Geometry: final body of the model. Coordinates: model frame, mm. Coordinates: 2 decimals unless noted, no trailing zeros. Order: outer loops, then holes, each group sorted by start corner. A loop starts at its lowest first (then second) coordinate and runs counter-clockwise, first axis right, second up. Notation, with made-up numbers: M 62,75.25 L 66,75.25 A24 cw 66,97.25 Z; hole C 80,67.25 d11. An arc over 180 degrees is marked long. One line per question, with ' | ' between items.
from build123d import *

# Parameters (mm, degrees)
F0_W     = 30
F0_H     = 34
F0_R     = 1.575
F1_DEPTH = 4.826
F2_R     = 5


with BuildPart() as f1:
    # F0 (on Top) → F1 (new body)
    with BuildSketch(Plane.XY):
        Rectangle(F0_W, F0_H)
        with Locations((-8.8, -10)):
            Circle(F0_R, mode=Mode.SUBTRACT)
        with Locations((8.8, -10)):
            Circle(F0_R, mode=Mode.SUBTRACT)
        with Locations((-8.8, 10)):
            Circle(F0_R, mode=Mode.SUBTRACT)
        with Locations((8.8, 10)):
            Circle(F0_R, mode=Mode.SUBTRACT)
    extrude(amount=F1_DEPTH)

    # F2
    f2_edges = [f1.edges().sort_by_distance(p)[0] for p in [
        (-15, -17, 2.413),
        (15, -17, 2.413),
        (-15, 17, 2.413),
        (15, 17, 2.413),
    ]]
    fillet(f2_edges, radius=F2_R)


solid = f1.part
1. Draft query along Y for faces 1 (the face through (10.255, 9.397, 2.379)), 2 (the face through (13, -16, 2)), 3 (the face through (15, 0, 2)). Return one class per face: pulls with the +Y half, pulls with the -Y half, needs draft (parallel to the pull), parting line crosses it, or undercut.
Response values:
face 1: undercut | face 2: pulls with the -Y half | face 3: needs draft
2. Section B-B, the plane y = 11. Output: boundary loops of the cut face in (x, z).
Response values:
outline: M -15,0 L -10.02,0 L -10.02,4.83 L -15,4.83 Z; M -7.58,0 L 7.58,0 L 7.58,4.83 L -7.58,4.83 Z; M 10.02,0 L 15,0 L 15,4.83 L 10.02,4.83 Z
3. Section A-A, the plane z = 1.7. Output: boundary loops of the cut face in (x, y) (3 decimals).
Response values:
outline: M -15,-12 A5 ccw -10,-17 L 10,-17 A5 ccw 15,-12 L 15,12 A5 ccw 10,17 L -10,17 A5 ccw -15,12 Z; hole C -8.8,-10 d3.15; hole C -8.8,10 d3.15; hole C 8.8,-10 d3.15; hole C 8.8,10 d3.15
4. Section C-C, the plane x = -8.8. Output: boundary loops of the cut face in (y, z) (3 decimals), and give its area (3 significant figures).
Response values:
outline: M -17,0 L -11.575,0 L -11.575,4.826 L -17,4.826 Z; M -8.425,0 L 8.425,0 L 8.425,4.826 L -8.425,4.826 Z; M 11.575,0 L 17,0 L 17,4.826 L 11.575,4.826 Z | area: 134 mm^2
5. Material intervals for line 1 (Y direction, x = 8.8, z = 1.2) (3 decimals); line 2 (Y direction, x = -9.5, z = 2.3); line 3 (Y direction, x = 13.5, z = 2.45), sorted ascending. Write a range as [from, to].
Response values:
line 1: y = [-17, -11.575], [-8.425, 8.425], [11.575, 17] | line 2: y = [-17, -11.41], [-8.59, 8.59], [11.41, 17] | line 3: y = [-15.57, 15.57]
